Input: part model. Units: mm. Frame: model coordinates. Face numbers are marked on the shaded views. A direction names the side the tool comes from. Coordinates: 2 decimals unless noted, no trailing zeros. Write each loop counter-clockwise with the first axis right and the second up, starting at its lowest first coordinate (ties: lowest second). Pieces come first, ordered by that corner, then holes. Notation, with made-up numbers: (86.25, 63) -> (104.25, 63) arc R14 cw to (104.25, 88) -> close; hole circle Ø10 at (87.25, 68). An arc over 180 degrees is marked (long way). Use one line per item in the form item = value. Start each with the question number.
(1) Cut plane D-D on z = 0.25. Return the cut outline in (x, y), plus the area to 3 significant figures.
(2) First-contact query: pin 1 (12 mm diameter, centred on x = 20.5, z = -1, fed in from -Y); pin 2 (12 mm diameter, centred on x = -15.5, z = -2, fed in from +Y) (3 decimals); pin 3 (3 mm diameter, centred on x = -10.5, y = 1, fed in from -Z). Flat tips, straight axial feed; report the tip coordinate or a pass-through.
(3) Cut plane A-A on z = -8. Return the cut outline in (x, y).
(4) Cut plane C-C on x = 21. Return the cut outline in (y, z).
(5) Ray query, line 1 along X through (y, z) = (1, -3); line 2 along Z through (x, y) = (-10, -4.25); line 3 along X through (y, z) = (1.5, -8). Return the intervals inside material, ascending.
(6) Set-up query: the marked faces 1, 2 and 3. Return all of +Z, -Z, +X, -X, +Y, -Y with unobstructed straight access to the full face (end or side cutting, diameter ignored); none if empty.
(7) Cut plane B-B on y = 1. Return the cut outline in (x, z), plus the area to 3 significant figures.
(8) Pull-direction query (Z, two-part tool) for the marked faces 4, 5 and 6; classes: released by +Z, released by -Z, zero draft, split by the parting line, or undercut.
Solid Edge part; units mm, degrees
sketch "Sketch1" plane through (0, 0, 0) normal (0, -1, 0) x (1, 0, 0)
  line L0 (-29.34, -10) -> (-25.34, -10)
  line L1 (-25.34, -10) -> (-25.34, 6)
  line L2 (-25.34, 6) -> (25.34, 6)
  line L3 (25.34, 6) -> (25.34, -10)
  line L4 (25.34, -10) -> (29.34, -10)
  line L5 (29.34, -10) -> (29.34, 10)
  line L6 (29.34, 10) -> (-29.34, 10)
  line L7 (-29.34, 10) -> (-29.34, -10)
  dimension "D1" = 25.34
  dimension "D2" = 29.34
  dimension "D3" = 29.34
  dimension "D4" = 25.34
extrude "Protrusion1" add sketch "Sketch1" along normal mid plane 10
sketch "Sketch2" plane through (0, 0, 0) normal (0, -1, 0) x (1, 0, 0)
  line L0 (-25.34, -10) -> (-25.34, -6)
  line L1 (-25.34, -6) -> (-22.84, -6)
  line L2 (-22.84, -6) -> (-25.34, -10)
  dimension "D1" = 25.34
  dimension "D2" = 25.34
extrude "ExtrudedProtrusion_3" add sketch "Sketch2" along normal mid plane 10
sketch "Sketch3" plane through (0, 0, 0) normal (0, -1, 0) x (1, 0, 0)
  line L0 (25.34, -10) -> (25.34, -6)
  line L1 (25.34, -6) -> (22.84, -6)
  line L2 (22.84, -6) -> (25.34, -10)
  dimension "D1" = 25.34
  dimension "D2" = 25.34
extrude "ExtrudedProtrusion_4" add sketch "Sketch3" along normal mid plane 10
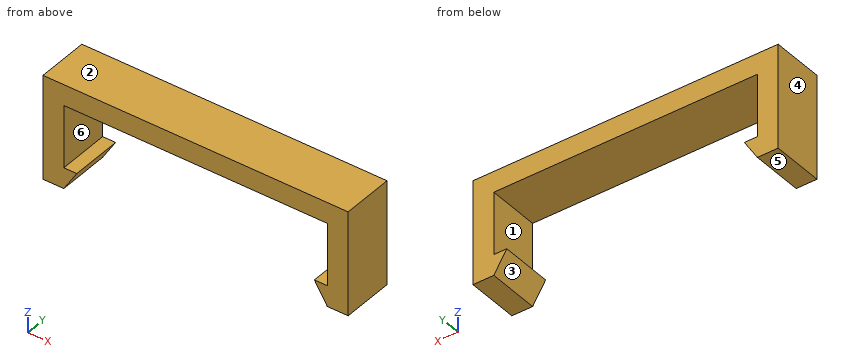
Values:
q1.outline = (-29.34, -5) -> (-25.34, -5) -> (-25.34, 5) -> (-29.34, 5) -> close; (25.34, -5) -> (29.34, -5) -> (29.34, 5) -> (25.34, 5) -> close
q1.area = 80.0 mm2
q2.pin_1 = -5
q2.pin_2 = through
q2.pin_3 = 6
q3.outline = (-29.34, -5) -> (-24.09, -5) -> (-24.09, 5) -> (-29.34, 5) -> close; (24.09, -5) -> (29.34, -5) -> (29.34, 5) -> (24.09, 5) -> close
q4.outline = (-5, 6) -> (5, 6) -> (5, 10) -> (-5, 10) -> close
q5.line_1 = -29.34 to -25.34, 25.34 to 29.34
q5.line_2 = 6 to 10
q5.line_3 = -29.34 to -24.09, 24.09 to 29.34
q6.face_1 = +Y, -Y
q6.face_2 = +Z, +X, -X, +Y, -Y
q6.face_3 = -Z, +Y, -Y
q7.outline = (-29.34, -10) -> (-25.34, -10) -> (-22.84, -6) -> (-25.34, -6) -> (-25.34, 6) -> (25.34, 6) -> (25.34, -6) -> (22.84, -6) -> (25.34, -10) -> (29.34, -10) -> (29.34, 10) -> (-29.34, 10) -> close
q7.area = 373 mm2
q8.face_4 = zero draft
q8.face_5 = released by -Z
q8.face_6 = undercut
